```python
from build123d import *

# Parameters (mm, degrees)
F0_R     = 112.5
F1_DEPTH = 4
F2_R     = 4.15
F3_DEPTH = 25
F4_R     = 112.5
F4_R_2   = 110.5
F5_DEPTH = 10


with BuildPart() as f1:
    # F0 (on Top) → F1 (new body)
    with BuildSketch(Plane.XY):
        Circle(F0_R)
    extrude(amount=F1_DEPTH)

    # F2 (on face) → F3 (cut)
    with BuildSketch(Plane.XY.offset(4)):
        with Locations((-74.2462, 74.2462)):
            Circle(F2_R)
        with Locations((-74.2462, -74.2462)):
            Circle(F2_R)
        with Locations((74.2462, -74.2462)):
            Circle(F2_R)
        with Locations((74.2462, 74.2462)):
            Circle(F2_R)
    extrude(amount=-F3_DEPTH, mode=Mode.SUBTRACT)

    # F4 (on face) → F5 (join)
    with BuildSketch(Plane.XY.offset(4)):
        Circle(F4_R)
        Circle(F4_R_2, mode=Mode.SUBTRACT)
    extrude(amount=F5_DEPTH)


solid = f1.part
```
Read the model definition and answer for the solid it produces. Units are mm, in the model's axes. A direction names the side the tool comes from. Give positions to 0.01 mm unless a question says otherwise; leave off trailing zeros. Write each loop counter-clockwise with the first axis right and the second up, starting at its lowest first coordinate (ties: lowest second). Pieces come first, ordered by that corner, then holes. Notation, with made-up numbers: (60.5, 20.25) -> (113.5, 20.25) arc R18 cw to (113.5, 36.25) -> close; hole circle Ø6 at (50, 26). An arc over 180 degrees is marked (long way). Answer in a Markdown table with one row per item.
1) Straight lines are drawn through the part: line 1 (Y direction, x = -72, z = 3.5); line 2 (X direction, y = 3, z = 7); line 3 (X direction, y = 72.5, z = 1.5). For each, find the intervals that lie inside material, in ascending order. Write a range as [from, to].
Results list:
| item | result |
|---|---|
| line 1 | [-86.44, -77.74], [-70.76, 70.76], [77.74, 86.44] |
| line 2 | [-112.46, -110.46], [110.46, 112.46] |
| line 3 | [-86.02, -78.01], [-70.48, 70.48], [78.01, 86.02] |
2) Determine the mould class of faces 1 (the cylindrical face through (-112.39, 4.95, 6.9)), 2 (the flat face through (83, -74, 14)), 3 (the cylindrical face through (78.08, -75.84, 2.03)) for opening direction Y: released by +Y, released by -Y, zero draft, split by the parting line, or undercut.
Results list:
| item | result |
|---|---|
| face 1 | split by the parting line |
| face 2 | zero draft |
| face 3 | undercut |
3) Each of these flat-tipped pins is pushed along its axis until it touches: pin 1 Ø5 at (x, y) = (-22.5, -86) entering from +Z; pin 2 Ø4 at (x, z) = (-11.5, 11) entering from -Y; pin 3 Ø8 at (y, z) = (-10.5, 7) entering from +X. Where does it stop, or does it pass through?
Results list:
| item | result |
|---|---|
| pin 1 | z = 4 |
| pin 2 | y = -112.1 |
| pin 3 | x = 112.31 |
4) Section C-C on z = 6.75 is taken. Give the vertices of the cut face in (x, y).
Results list:
| item | result |
|---|---|
| outline | circle Ø225 at (0, 0); hole circle Ø221 at (0, 0) |
5) Section A-A on y = 0 is taken. Give the vertices of the cut face in (x, z), plus the area to 3 significant figures.
Results list:
| item | result |
|---|---|
| outline | (-112.5, 0) -> (112.5, 0) -> (112.5, 14) -> (110.5, 14) -> (110.5, 4) -> (-110.5, 4) -> (-110.5, 14) -> (-112.5, 14) -> close |
| area | 940 mm^2 |
6) A tool of negligible diameter and unlimited length cuts with its end or side. For faces 4 (the cylindrical face through (-72.331, 70.564, 2.028)), 5 (the cylindrical face through (-23.954, -107.872, 8.93)), from which of +Z, -Z, +X, -X, +Y, -Y can it reach the whole face along a straight path? Write none if from no direction.
Results list:
| item | result |
|---|---|
| face 4 | +Z, -Z |
| face 5 | +Z |
